Design review of the part built by this model. Coordinates are the model's own, in mm. A direction names the side the tool comes from. Coordinates: 2 decimals unless noted, no trailing zeros. Loops run counter-clockwise (first coordinate to the right, second up) from the corner with the lowest first, then second, coordinate; pieces in that order, holes last. Notation, with made-up numbers: (-39.75, 33) -> (-31.75, 33) arc R36 cw to (-31.75, 71) -> close; hole circle Ø11 at (-8.75, 85.25). An arc over 180 degrees is marked (long way). One line per item, written item: value. Start each with the question number.
1. Machinability: for faces 1 (the flat face through (6.35, 12, -5)), 2 (the flat face through (19.05, 16, -17)), 3 (the flat face through (0, 19.05, -21)), 4 (the flat face through (0.27, 12.7, -19.23)), which of the approach directions +Z, -Z, +X, -X, +Y, -Y give a long, thin tool a straight path to every point of the face, cutting with its end or side? Answer none if there is none.
2. Add section B-B on y = 2. Write out the cut boundary in (x, z), plus the area to 3 significant figures.
3. Add section C-C on x = 15.5. Write out the cut boundary in (y, z), plus the area to 3 significant figures.
4. Draft analysis for pull direction X (two halves, no side actions). For faces 5 (the flat face through (-19.05, 16, -17)), 6 (the flat face through (0, 16, -19.05)), 7 (the flat face through (-13, 9, 0)), state which applies: pulls with the +X half, pulls with the -X half, needs draft (parallel to the pull), parting line crosses it, or undercut.
5. Insertion check: pin 1 (1.5 mm diameter, centred on x = 11.5, z = -21, fed in from +Y); pin 2 (4 mm diameter, centred on x = 0.5, y = 22.5, fed in from +Z); pin 3 (1.9 mm diameter, centred on x = 2, y = 16.5, fed in from +Z). Each pin has a flat end and moves straight along its axis. Give the tip position at first contact, or say it passes through.
6. Add section D-D on y = 30.5. Write out the cut boundary in (x, z), plus the area to 3 significant figures.
7. Add section A-A on z = -10. Write out the cut boundary in (x, y), plus the area to 3 significant figures.
8. For probe 1 along X at (y, z) = (17, -12); probe 2 along Y at (x, z) = (12, -30), list the stretches that pass through material, from the lowest coordinate up.
```python
from build123d import *

# Parameters (mm, degrees)
BOSS_EXTRUDE1_DEPTH     = 19.05
CUT_EXTRUDE1_DEPTH      = 38.1
CUT_EXTRUDE1_DEPTH_BACK = 42.639734629
SKETCH2_W               = 12.7
SKETCH2_H               = 19.05


with BuildPart() as part:
    # Sketch1 → Boss-Extrude1 (new, symmetric)
    with BuildSketch(Plane(origin=(0, 0, 0), x_dir=(0, 0, -1), z_dir=(1, 0, 0))):
        Polygon((0, 0), (0, 19.05), (25.4, 19.05), (25.4, 31.75), (31.75, 31.75), (31.75, 12.7), (6.35, 12.7), (6.35, 0), align=None)
    extrude(amount=BOSS_EXTRUDE1_DEPTH, both=True)

    # Sketch2 → Cut-Extrude1 (cut, two sides: drawn at the far end of the back side and taken through both)
    with BuildSketch(Plane(origin=(0, 19.05, 0), x_dir=(1, 0, 0), z_dir=(0, 1, 0)).offset(-CUT_EXTRUDE1_DEPTH_BACK)):
        with Locations((0, 9.525)):
            Rectangle(SKETCH2_W, SKETCH2_H)
    extrude(amount=CUT_EXTRUDE1_DEPTH + CUT_EXTRUDE1_DEPTH_BACK, mode=Mode.SUBTRACT)


solid = part.part
```
Worked answers:
1. face 1: +Z, +Y, -Y
1. face 2: +Z, -Z, +X, +Y, -Y
1. face 3: +Z, +X, -X, +Y
1. face 4: -Z, +X, -X, -Y
2. outline: (-19.05, -6.35) -> (-6.35, -6.35) -> (-6.35, 0) -> (-19.05, 0) -> close; (6.35, -6.35) -> (19.05, -6.35) -> (19.05, 0) -> (6.35, 0) -> close
2. area: 161 mm²
3. outline: (0, -6.35) -> (12.7, -6.35) -> (12.7, -31.75) -> (31.75, -31.75) -> (31.75, -25.4) -> (19.05, -25.4) -> (19.05, 0) -> (0, 0) -> close
3. area: 363 mm²
4. face 5: pulls with the -X half
4. face 6: undercut
4. face 7: needs draft
5. pin 1: stops at y = 19.05
5. pin 2: stops at z = -25.4
5. pin 3: stops at z = -19.05
6. outline: (-19.05, -31.75) -> (19.05, -31.75) -> (19.05, -25.4) -> (-19.05, -25.4) -> close
6. area: 242 mm²
7. outline: (-19.05, 12.7) -> (-6.35, 12.7) -> (-6.35, 19.05) -> (-19.05, 19.05) -> close; (6.35, 12.7) -> (19.05, 12.7) -> (19.05, 19.05) -> (6.35, 19.05) -> close
7. area: 161 mm²
8. probe 1: x = -19.05 to -6.35, 6.35 to 19.05
8. probe 2: y = 12.7 to 31.75
